The model under review builds one solid part; all positions refer to its coordinate system, in mm. A direction names the side the tool comes from. Round coordinates to 2 decimals unless told otherwise and drop trailing zeros. Write each loop counter-clockwise with the first axis right and the second up, starting at its lowest first coordinate (ties: lowest second). Pieces come first, ordered by that corner, then holes. Notation, with made-up numbers: (22, 1) -> (31, 1) arc R11 ccw to (31, 22) -> close; hole circle Ø4 at (19, 39). An arc over 180 degrees is marked (long way). Return JSON: item names as keys, results as strings. Group by question number.
1. Take a section at A-A, the plane y = 16.5. Write out the cut boundary in (x, z) (3 decimals).
2. Take a section at D-D, the plane y = 8. Write out the cut boundary in (x, z) (3 decimals), then the cut area to 3 significant figures.
3. Mouldability with a two-part tool opening along Z and no side actions: class faces 1 (the flat face through (16, 4, 5)), 2 (the flat face through (0, 0, -25)), 3 (the flat face through (-10, 7, 8.25)) as pulls with the +Z half, pulls with the -Z half, needs draft (parallel to the pull), parting line crosses it, or undercut.
4. Take a section at B-B, the plane z = 6. Write out the cut boundary in (x, y).
5. Clearance check with flat-ended pins moving along their axes: P1, Ø1.1, axis at x = -10.5, y = 5.5, coming from the -Z side; P2, Ø8, axis at y = -9.5, z = -1, coming from the -X side; P3, Ø3, axis at x = 4, y = 1, coming from the +Z side; P4, Ø6, axis at x = 0.5, y = 8.5, coming from the -Z side. State where each tip first meets the part, or that it passes through.
6. For line 1 along X through (y, z) = (19, 6); line 2 along Z through (x, y) = (-5, 11.5); line 3 along Y through (x, z) = (-8, 8), list the stretches that pass through material, from the lowest coordinate up. Write a range as from..to.
7. Tool access review of faces 4 (the cylindrical face through (0.867, -3.905, -12.353)), 5 (the flat face through (9.125, 7, 9)), 6 (the flat face through (11.25, 7, 7)): name each direction out of +Z, -Z, +X, -X, +Y, -Y from which nothing blocks a thin tool from reaching the whole face with its end or side.
8. Take a section at C-C, the plane x = 8. Write out the cut boundary in (y, z), then the cut area to 3 significant figures.
from build123d import *

# Parameters (mm, degrees)
SKETCH1_W               = 32
SKETCH1_H               = 27
BOSS_EXTRUDE1_DEPTH     = 10
SKETCH3_R               = 4
BOSS_EXTRUDE2_DEPTH     = 25
SKETCH4_W               = 32
SKETCH4_H               = 10
BOSS_EXTRUDE3_DEPTH     = 8
CUT_EXTRUDE4_DEPTH      = 9
CUT_EXTRUDE4_DEPTH_BACK = 21
SKETCH6_W               = 2.4
SKETCH6_H               = 32
FILLET1_R               = 2


with BuildPart() as part:
    # Sketch1 → Boss-Extrude1 (new body)
    with BuildSketch(Plane.XY):
        Rectangle(SKETCH1_W, SKETCH1_H)
    extrude(amount=BOSS_EXTRUDE1_DEPTH)

    # Sketch3 → Boss-Extrude2 (add)
    with BuildSketch(Plane(origin=(0, 0, 0), x_dir=(-1, 0, 0), z_dir=(0, 0, -1))):
        Circle(SKETCH3_R)
    extrude(amount=BOSS_EXTRUDE2_DEPTH)


with BuildPart() as body_2:
    # Sketch4 → Boss-Extrude3 (new body)
    with BuildSketch(Plane(origin=(0, 13.5, 0), x_dir=(1, 0, 0), z_dir=(0, 1, 0))):
        with Locations((0, -5)):
            Rectangle(SKETCH4_W, SKETCH4_H)
    extrude(amount=BOSS_EXTRUDE3_DEPTH)


with BuildPart() as cut_extrude4_tool:
    # Sketch2 → Cut-Extrude4 (new body, two sides)
    with BuildSketch(Plane(origin=(0, 13.5, 0), x_dir=(1, 0, 0), z_dir=(0, 1, 0))) as cut_extrude4_sk:
        Polygon((-9.125, -10), (-9.125, -8.25), (-11.25, -8.25), (-11.25, -5), (11.25, -5), (11.25, -8.25), (9.125, -8.25), (9.125, -10), align=None)
    extrude(amount=CUT_EXTRUDE4_DEPTH)
    extrude(cut_extrude4_sk.sketch, amount=-CUT_EXTRUDE4_DEPTH_BACK)


with BuildPart() as part_1:
    add(part.part)

    # Cut-Extrude4: cut by cut_extrude4_tool
    add(cut_extrude4_tool.part, mode=Mode.SUBTRACT)


with BuildPart() as body_2_1:
    add(body_2.part)

    # Cut-Extrude4: cut by cut_extrude4_tool
    add(cut_extrude4_tool.part, mode=Mode.SUBTRACT)

    # Sketch6 → M4 Clearance Hole1 (revolve, cut)
    with BuildSketch(Plane(origin=(-16, 16.5, 5), x_dir=(0, 0, 1), z_dir=(0, 1, 0))):
        with Locations((1.2, 16)):
            Rectangle(SKETCH6_W, SKETCH6_H)
    revolve(axis=Axis((-22.35, 16.5, 5), (1, 0, 0)), mode=Mode.SUBTRACT)

    # Combine1: union part
    add(part_1.part)

    # Fillet1
    fillet1_edges = [body_2_1.edges().sort_by_distance(p)[0] for p in [
        (16, 21.5, 5),
        (-16, 21.5, 5),
        (-16, -13.5, 5),
        (16, -13.5, 5),
        (4, 0, 0),
        (4, 0, -25),
    ]]
    fillet(fillet1_edges, radius=FILLET1_R)


solid = body_2_1.part
Output:
{
 "1": {"outline": "(-16, 0) -> (16, 0) -> (16, 2.6) -> (-16, 2.6) -> close; (-16, 7.4) -> (-11.25, 7.4) -> (-11.25, 8.25) -> (-9.125, 8.25) -> (-9.125, 10) -> (-16, 10) -> close; (9.125, 8.25) -> (11.25, 8.25) -> (11.25, 7.4) -> (16, 7.4) -> (16, 10) -> (9.125, 10) -> close"},
 "2": {"outline": "(-16, 0) -> (16, 0) -> (16, 10) -> (9.125, 10) -> (9.125, 8.25) -> (11.25, 8.25) -> (11.25, 5) -> (-11.25, 5) -> (-11.25, 8.25) -> (-9.125, 8.25) -> (-9.125, 10) -> (-16, 10) -> close", "area": "215 mm^2"},
 "3": {"face 1": "needs draft", "face 2": "pulls with the -Z half", "face 3": "undercut"},
 "4": {"outline": "(-16, -11.5) arc R2 ccw to (-14, -13.5) -> (14, -13.5) arc R2 ccw to (16, -11.5) -> (16, 14.32) -> (11.25, 14.32) -> (11.25, -7.5) -> (-11.25, -7.5) -> (-11.25, 14.32) -> (-16, 14.32) -> close; (-16, 18.68) -> (-11.25, 18.68) -> (-11.25, 21.5) -> (-14, 21.5) arc R2 ccw to (-16, 19.5) -> close; (11.25, 18.68) -> (16, 18.68) -> (16, 19.5) arc R2 ccw to (14, 21.5) -> (11.25, 21.5) -> close"},
 "5": {"P1": "stops at z = 0", "P2": "stops at x = -16", "P3": "stops at z = 5", "P4": "stops at z = -0.06"},
 "6": {"line 1": "x = -16..-11.25, 11.25..16", "line 2": "z = 0..5", "line 3": "y = -13.5..-7.5"},
 "7": {"face 4": "-Z", "face 5": "+Z, +Y", "face 6": "+Y"},
 "8": {"outline": "(-13.5, 0) -> (21.5, 0) -> (21.5, 5) -> (18.9, 5) arc R2.4 cw to (14.1, 5) -> (-7.5, 5) -> (-7.5, 10) -> (-13.5, 10) -> close", "area": "196 mm^2"}
}
